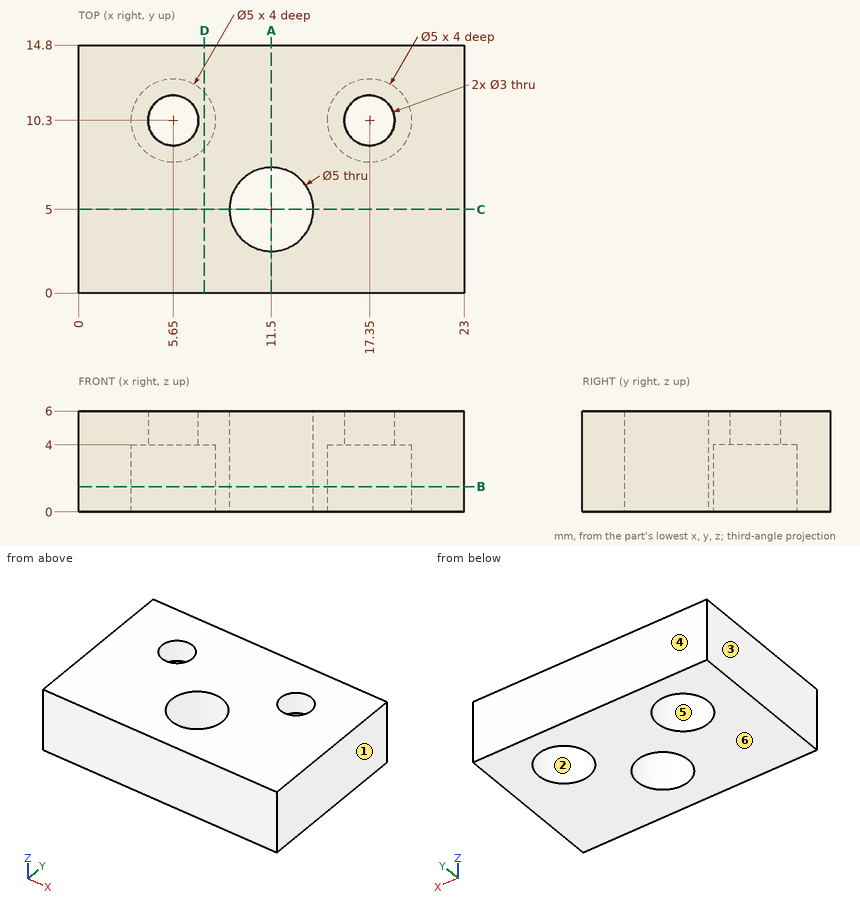
Geometry: see drawing. Coordinates: mm, zero at the bounding-box minimum. A direction names the side the tool comes from. Give positions to 0.01 mm unless a question says otherwise; leave off trailing zeros. Loops run counter-clockwise (first coordinate to the right, second up) from the corner with the lowest first, then second, coordinate; pieces in that order, holes last. Notation, with made-up numbers: M 52.25,55.25 L 94.25,55.25 A13 ccw 94.25,61.25 Z; hole C 60,24.25 d9. An arc over 180 degrees is marked long. Answer as CSV lines item,"result". Start each with the question number.
1. Section B-B on z = 1.5. Return loops of the section in (x, y), plus the area to 3 significant figures.
2. Section C-C on y = 5. Return loops of the section in (x, z), plus the area to 3 significant figures.
3. Pull-direction query (X, two-part tool) for the marked faces 1, 2, 3 and 4; classes: released by +X, released by -X, zero draft, split by the parting line, or undercut.
4. Section A-A on x = 11.5. Return loops of the section in (y, z).
5. Section D-D on x = 7.5. Return loops of the section in (y, z).
6. Reachability of the marked faces 5 and 6 from +Z, -Z, +X, -X, +Y, -Y: full face, straight path, thin tool, end or side. Return the list, or none.
7. Pin query (flat end, axial travel): P1, Ø4.5, axis at x = 17.35, y = 10.3, coming from the -Z side. Return the tip coordinate at first contact, or that it passes through.
8. Line query: L1, parallel to X at y = 10.3, z = 4.7; L2, parallel to Y at x = 11.5, z = 2.7; L3, parallel to Y at x = 5.65, z = 2.15. Output: solid intervals per line, ascending.
Computed values:
1,outline,"M 0,0 L 23,0 L 23,14.8 L 0,14.8 Z; hole C 5.65,10.3 d5; hole C 11.5,5 d5; hole C 17.35,10.3 d5"
1,area,"281 mm²"
2,outline,"M 0,0 L 9,0 L 9,6 L 0,6 Z; M 14,0 L 23,0 L 23,6 L 14,6 Z"
2,area,"108 mm²"
3,face 1,"released by +X"
3,face 2,"undercut"
3,face 3,"released by -X"
3,face 4,"zero draft"
4,outline,"M 0,0 L 2.5,0 L 2.5,6 L 0,6 Z; M 7.5,0 L 14.8,0 L 14.8,6 L 7.5,6 Z"
5,outline,"M 0,0 L 8.62,0 L 8.62,4 L 11.98,4 L 11.98,0 L 14.8,0 L 14.8,6 L 0,6 Z"
6,face 5,"-Z"
6,face 6,"-Z, +X, -X, +Y, -Y"
7,P1,"stops at z = 4"
8,L1,"x = 0 to 4.15, 7.15 to 15.85, 18.85 to 23"
8,L2,"y = 0 to 2.5, 7.5 to 14.8"
8,L3,"y = 0 to 7.8, 12.8 to 14.8"
